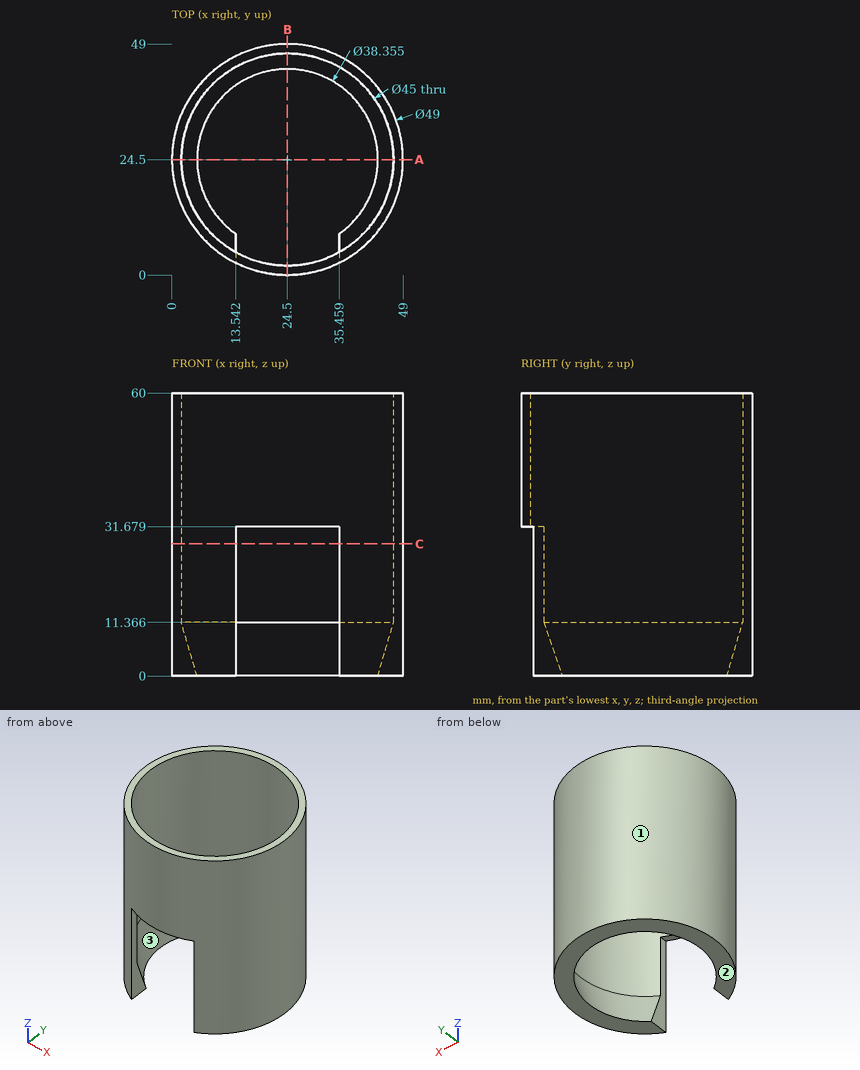
Design review of the part shown in the three views and the two pictorial views. Dimensions are in mm from the part's minimum x, y and z. Round coordinates to 2 decimals unless told otherwise and drop trailing zeros. Loops run counter-clockwise (first coordinate to the right, second up) from the corner with the lowest first, then second, coordinate; pieces in that order, holes last.
Q1. Add section C-C on z = 28. Write out the cut boundary in (x, y), plus the area to 3 significant figures.
Result sheet:
outline: (13.54, 2.59) - (13.54, 4.85) arc R22.5 cw (long way) to (35.46, 4.85) - (35.46, 2.59) arc R24.5 ccw (long way) to start
area: 250 mm2
Q2. Mouldability with a two-part tool opening along Y and no side actions: class the marked faces 1, 2 and 3 as +Y half, -Y half, draft (parallel to the pull), parting line (faces both ways), or undercut.
Result sheet:
face 1: parting line
face 2: draft
face 3: undercut
Q3. Add section A-A on y = 24.5. Write out the cut boundary in (x, z).
Result sheet:
outline: (0, 0) - (5.32, 0) - (2, 11.37) - (2, 60) - (0, 60) - close; (43.68, 0) - (49, 0) - (49, 60) - (47, 60) - (47, 11.37) - close
Q4. To check wall thickness, follow line 1 along X through (y, z) = (24.5, 40.5); line 2 along X through (y, z) = (12, 44.5). State the ranges of each line that lie inside material, in increasing order.
Result sheet:
line 1: x = 0 to 2, 47 to 49
line 2: x = 3.43 to 5.79, 43.21 to 45.57
Q5. Add section B-B on x = 24.5. Write out the cut boundary in (y, z).
Result sheet:
outline: (0, 31.68) - (2, 31.68) - (2, 60) - (0, 60) - close; (43.68, 0) - (49, 0) - (49, 60) - (47, 60) - (47, 11.37) - close
Q6. Insertion check: pin 1 Ø12 at (y, z) = (14, 30) entering from +X; pin 2 Ø6 at (x, z) = (27.5, 31) entering from -Y; pin 3 Ø4 at (x, y) = (20, 2.5) entering from -Z; pin 4 Ø8 at (x, y) = (20, 11) entering from +Z. Each pin has a flat end and moves straight along its axis. Give the tip position at first contact, or say it passes through.
Result sheet:
pin 1: stops at x = 48.58
pin 2: stops at y = 0
pin 3: stops at z = 31.68
pin 4: passes through
